Design review of the part built by this model. Coordinates are the model's own, in mm. A direction names the side the tool comes from. Round coordinates to 2 decimals unless told otherwise and drop trailing zeros. Order: outer loops, then holes, each group sorted by start corner. A loop starts at its lowest first (then second) coordinate and runs counter-clockwise, first axis right, second up. Notation, with made-up numbers: M 80,54 L 120,54 A25 cw 120,71 Z; hole C 73.25,0 d9. An arc over 180 degrees is marked long. Write each question's results on one line, items separated by ' | '. Start each with the question number.
Item 1: The part is to be moulded in two halves that separate along X. For faces 4 (the flat face through (-9.9, 1.48, 8.77)), 5 (the cylindrical face through (-52.43, 1.52, 9.4)), 6 (the flat face through (-22, 0, 0)), say which applies: +X half, -X half, draft (parallel to the pull), parting line (faces both ways), or undercut.
Item 2: Take a section at A-A, the plane x = 4. Write out the cut boundary in (y, z), plus the area to 3 significant figures.
Item 3: Wall thickness on line 1 (Z direction, x = -15.5, y = 2.6); line 2 (X direction, y = 1.25, z = 0.25); line 3 (Z direction, x = 5, y = 2.25): over which ranges is each line inside the solid? List them lowest first. Write a range as [from, to].
Item 4: Take a section at B-B, the plane z = -1.75. Write out the cut boundary in (x, y), plus the area to 3 significant figures.
Item 5: Take a section at C-C, the plane y = 2.3. Write out the cut boundary in (x, z).
Item 6: Machinability: for faces 1 (the flat face through (-9.836, 1.479, -8.732)), 2 (the flat face through (-31, 1, -10)), 3 (the flat face through (3.585, 1.521, -3.486)), which of the approach directions +Z, -Z, +X, -X, +Y, -Y give a long, thin tool a straight path to every point of the face, cutting with its end or side? Answer none if there is none.
Item 7: Take a section at D-D, the plane x = -27. Write out the cut boundary in (y, z), plus the area to 3 significant figures.
Item 8: Clearance check with a flat-ended pin moving along its axis: pin 1 (1 mm diameter, centred on x = 3.5, y = 2, fed in from -Z). State where the tip first meets the part, or that it passes through.
```python
from build123d import *

# Parameters (mm, degrees)
EXTRUDE_1_DEPTH     = 3
FILLET_1_R          = 2
CUT_EXTRUDE_1_DEPTH = 55.162371625


with BuildPart() as part:
    # 草图2 → 凸台-拉伸1 (new body)
    with BuildSketch(Plane(origin=(0, 0, 0), x_dir=(1, 0, 0), z_dir=(0, 1, 0))):
        with BuildLine():
            Line((-12.031587919, -10), (-7.7014609, -7.5))
            ThreePointArc((-7.7014609, -7.5), (10.75, 0), (-7.7014609, 7.5))
            Line((-7.7014609, 7.5), (-12.031587919, 10))
            Line((-12.031587919, 10), (-53, 10))
            Line((-53, 10), (-53, -10))
            Line((-53, -10), (-12.031587919, -10))
        make_face()
    extrude(amount=EXTRUDE_1_DEPTH)

    # 圆角1
    fillet_1_edges = [part.edges().sort_by_distance(p)[0] for p in [
        (-53, 1.5, -10),
        (-53, 1.5, 10),
    ]]
    fillet(fillet_1_edges, radius=FILLET_1_R)

    # 草图3 → 切除-拉伸1 (cut, through all)
    with BuildSketch(Plane(origin=(0, 3, 0), x_dir=(1, 0, 0), z_dir=(0, 1, 0))):
        Polygon((0, 7.071067812), (-7.071067812, 0), (0, -7.071067812), (7.071067812, 0), align=None)
    extrude(amount=-CUT_EXTRUDE_1_DEPTH, mode=Mode.SUBTRACT)


solid = part.part
```
Results list:
1) face 4: undercut | face 5: -X half | face 6: draft
2) outline: M 0,-9.98 L 3,-9.98 L 3,-3.07 L 0,-3.07 Z; M 0,3.07 L 3,3.07 L 3,9.98 L 0,9.98 Z | area: 41.4 mm²
3) line 1: [-10, 10] | line 2: [-53, -6.82], [6.82, 10.75] | line 3: [-9.52, -2.07], [2.07, 9.52]
4) outline: M -53,0 L -5.32,0 L -5.32,3 L -53,3 Z; M 5.32,0 L 10.61,0 L 10.61,3 L 5.32,3 Z | area: 159 mm²
5) outline: M -53,-8 A2 ccw -51,-10 L -12.03,-10 L -7.7,-7.5 A10.75 ccw long -7.7,7.5 L -12.03,10 L -51,10 A2 ccw -53,8 Z; hole M -7.07,0 L 0,-7.07 L 7.07,0 L 0,7.07 Z
6) face 1: -Z, +Y, -Y | face 2: -Z, -X, +Y, -Y | face 3: +Y, -Y
7) outline: M 0,-10 L 3,-10 L 3,10 L 0,10 Z | area: 60.0 mm²
8) pin 1: z = -10.32
